Geometry: final body of the model. Coordinates: model frame, mm. Face numbers are marked on the shaded views. A direction names the side the tool comes from. Give positions to 0.01 mm unless a question says otherwise; leave off trailing zeros. Order: outer loops, then holes, each group sorted by start corner. A loop starts at its lowest first (then second) coordinate and runs counter-clockwise, first axis right, second up. Notation, with made-up numbers: (13, 9) -> (30, 9) arc R32 ccw to (30, 47) -> close; hole circle Ø5 at (21, -9.75). An arc over 180 degrees is marked (long way). One line per question, with ' | ' between items.
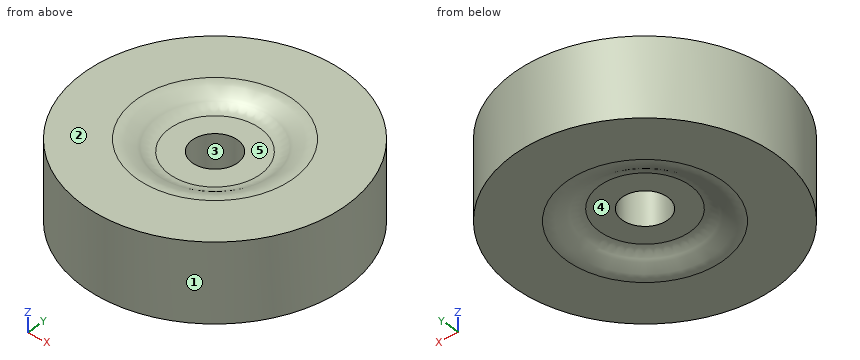
from build123d import *

# Parameters (mm, degrees)
F0_W = 12.8
F0_H = 19


with BuildPart() as f1:
    # F0 (on Front) → F1 (revolve)
    with BuildSketch(Plane.XZ):
        with BuildLine():
            Line((11, 6.625), (5.5, 6.625))
            Line((5.5, 6.625), (5.5, -6.625))
            Line((5.5, -6.625), (11, -6.625))
            add(Edge.make_bspline(
                [(11, -6.625), (12.4770218782, -6.8073266533), (13.8361511082, -7.7060788567), (14.2416545495, -8.0680834721), (16.9917661697, -9.7409561276), (19, -9.5)],
                knots=[0, 0, 0, 0, 0.3689001328, 0.5280858278, 1, 1, 1, 1], degree=3))
            Line((19, -9.5), (19, 9.5))
            add(Edge.make_bspline(
                [(11, 6.625), (12.4770218782, 6.8073266533), (13.8361511082, 7.7060788567), (14.2416545495, 8.0680834721), (16.9917661697, 9.7409561276), (19, 9.5)],
                knots=[0, 0, 0, 0, 0.3689001328, 0.5280858278, 1, 1, 1, 1], degree=3))
        make_face()
        with Locations((25.4, 0)):
            Rectangle(F0_W, F0_H)
    revolve(axis=Axis((0, 0, -0.4735022907), (0, 0, -1)))


solid = f1.part
1) Section B-B on y = 21.5. Return loops of the section in (x, z), plus the area to 3 significant figures.
Check result:
outline: (-23.43, -9.5) -> (23.43, -9.5) -> (23.43, 9.5) -> (-23.43, 9.5) -> close | area: 890 mm^2
2) Pull-direction query (Y, two-part tool) for the marked faces 1, 2 and 3; classes: +Y half, -Y half, draft (parallel to the pull), parting line (faces both ways), or undercut.
Check result:
face 1: parting line | face 2: draft | face 3: undercut
3) Section C-C on x = 28. Return loops of the section in (y, z), plus the area to 3 significant figures.
Check result:
outline: (-15.07, -9.5) -> (15.07, -9.5) -> (15.07, 9.5) -> (-15.07, 9.5) -> close | area: 573 mm^2
4) Material intervals for probe 1 along Y at (x, z) = (0, 2.25); probe 2 along Z at (x, y) = (-16.5, 20), sorted ascending. Write a range as from..to.
Check result:
probe 1: y = -31.8..-5.5, 5.5..31.8 | probe 2: z = -9.5..9.5
5) Set-up query: the marked faces 4 and 5. Return all of +Z, -Z, +X, -X, +Y, -Y with unobstructed straight access to the full face (end or side cutting, diameter ignored); none if empty.
Check result:
face 4: -Z | face 5: +Z
6) Section A-A on z = 0.25. Return loops of the section in (x, y).
Check result:
outline: circle Ø63.6 at (0, 0); hole circle Ø11 at (0, 0)
7) Contact query for flat-ended pins moving along their axis: pin 1 Ø2 at (x, z) = (-25, -7.5) entering from -Y; pin 2 Ø14.5 at (x, y) = (0, 0) entering from +Z (3 decimals); pin 3 Ø5 at (x, y) = (15, 8.5) entering from -Z; pin 4 Ø11 at (x, y) = (1.5, 3.5) entering from -Z (3 decimals). Output: stop coordinate, or through.
Check result:
pin 1: stops at y = -20.86 | pin 2: stops at z = 6.625 | pin 3: stops at z = -9.53 | pin 4: stops at z = -6.625
